from build123d import *

# Parameters (mm, degrees)
PAD_DEPTH          = 6.35
POCKET_DEPTH       = 930.254973
POLARPATTERN_COUNT = 18
POLARPATTERN_ANGLE = 66


with BuildPart() as part:
    # Sketch001 → Pad (new body)
    with BuildSketch(Plane.XZ.offset(9.652)):
        with BuildLine():
            Line((-225.298, 381), (225.298, 381))
            Line((225.298, 381), (225.298, 279.4))
            Line((225.298, 279.4), (195.637986, 279.4))
            ThreePointArc((195.637986, 279.4), (0, 341.08442), (-195.637986, 279.4))
            Line((-225.298, 279.4), (-195.637986, 279.4))
            Line((-225.298, 279.4), (-225.298, 381))
        make_face()
    extrude(amount=PAD_DEPTH)

    # Sketch002 (on Face8 of Pad) → Pocket (cut, through all)
    with BuildSketch(Plane.XZ.offset(16.002)):
        with BuildLine():
            Line((-168.490483, 291.336334), (-190.854721, 293.415253))
            Line((-190.854721, 293.415253), (-198.020414, 272.128312))
            ThreePointArc((-168.490483, 291.336334), (-183.506939, 282.118957), (-198.020414, 272.128312))
        make_face()
    pocket = extrude(amount=-POCKET_DEPTH, mode=Mode.SUBTRACT)

    # PolarPattern: Pocket ×18 about axis
    polarpattern_axis = Axis((0, 0, 0), (0, 1, 0))
    for i in range(1, POLARPATTERN_COUNT):
        add(pocket.rotate(polarpattern_axis, i * POLARPATTERN_ANGLE / (POLARPATTERN_COUNT - 1)), mode=Mode.SUBTRACT)


solid = part.part
Design review of the part built by this model. Coordinates are the model's own, in mm. A direction names the side the tool comes from. Give positions to 0.01 mm unless a question says otherwise; leave off trailing zeros. Loops run counter-clockwise (first coordinate to the right, second up) from the corner with the lowest first, then second, coordinate; pieces in that order, holes last. Notation, with made-up numbers: M 15.25,-5 L 36.25,-5 A23 cw 36.25,30 Z; hole C -18.5,23 d7. An arc over 180 degrees is marked long. Answer as a JSON object with one key per item and string values.
Item 1: We need section B-B (x = -27.5). State the section outline as (y, z) points.
Output values:
{"outline": "M -16,342.93 L -9.65,342.93 L -9.65,381 L -16,381 Z"}
Item 2: Mouldability with a two-part tool opening along X and no side actions: class faces 3 (the face through (29.14, -12.871, 344.337)), 4 (the face through (3, -9.652, 353)) as pulls with the +X half, pulls with the -X half, needs draft (parallel to the pull), parting line crosses it, or undercut.
Output values:
{"face 3": "undercut", "face 4": "needs draft"}
Item 3: Machinability: for faces 1 (the face through (3, -16.002, 353)), 2 (the face through (-29.5, -12.9, 344.2)), which of the approach directions +Z, -Z, +X, -X, +Y, -Y give a long, thin tool a straight path to every point of the face, cutting with its end or side? Answer none if there is none.
Output values:
{"face 1": "+Z, -Z, +X, -X, -Y", "face 2": "-Z, +Y, -Y"}
Item 4: We need section A-A (x = 186.5). State the section outline as (y, z) points, and give its area (3 significant figures).
Output values:
{"outline": "M -16,293.33 L -9.65,293.33 L -9.65,381 L -16,381 Z", "area": "557 mm2"}
Item 5: Wall thickness on line 1 along X through (y, z) = (-15.5, 348); line 2 along Z through (x, y) = (22, -13.5); line 3 along X through (y, z) = (-12.75, 349): over which ranges is each line inside the solid? List them lowest first.
Output values:
{"line 1": "x = -225.3 to -35.97, -35.47 to -14.25, -9.65 to 9.12, 13.76 to 34.87, 35.51 to 225.3", "line 2": "z = 341.03 to 381", "line 3": "x = -225.3 to -13.08, -11.01 to 10.47, 12.58 to 225.3"}
